For this review, use the dimensioned drawing (mm, ordinates from the lowest corner) and the shaded views. Give positions to 0.01 mm unless a question says otherwise; leave off trailing zeros. Order: outer loops, then holes, each group sorted by start corner. A loop starts at its lowest first (then second) coordinate and runs counter-clockwise, first axis right, second up. Notation, with made-up numbers: M 62,81 L 120,81 A10 cw 120,86 Z; hole C -32.5,23.25 d6. An arc over 180 degrees is marked long. Answer as CSV lines item,"result". Start each with the question number.
1. We need section B-B, the plane x = 114.3. Give the boundary of the cut face in (y, z) (3 decimals).
2. We need section C-C, the plane y = 50.8. Give the boundary of the cut face in (x, z) (3 decimals).
3. Clearance check with flat-ended pins moving along their axes: P1, Ø4, axis at x = 31.75, y = 50.8, coming from the -Z side; P2, Ø6, axis at x = 31.75, y = 12.7, coming from the +Z side (3 decimals). State where each tip first meets the part, or that it passes through.
4. We need section D-D, the plane y = 33. Give the boundary of the cut face in (x, z) (3 decimals), and give its area (3 significant figures).
5. We need section A-A, the plane x = 63.5. Give the boundary of the cut face in (y, z) (1 decimal), and give its area (3 significant figures).
6. For line 1 along Y through (x, z) = (12.7, 1.55); line 2 along X through (y, z) = (50.8, 1.1); line 3 along X through (y, z) = (12, 2.65), list the stretches that pass through material, from the lowest coordinate up.
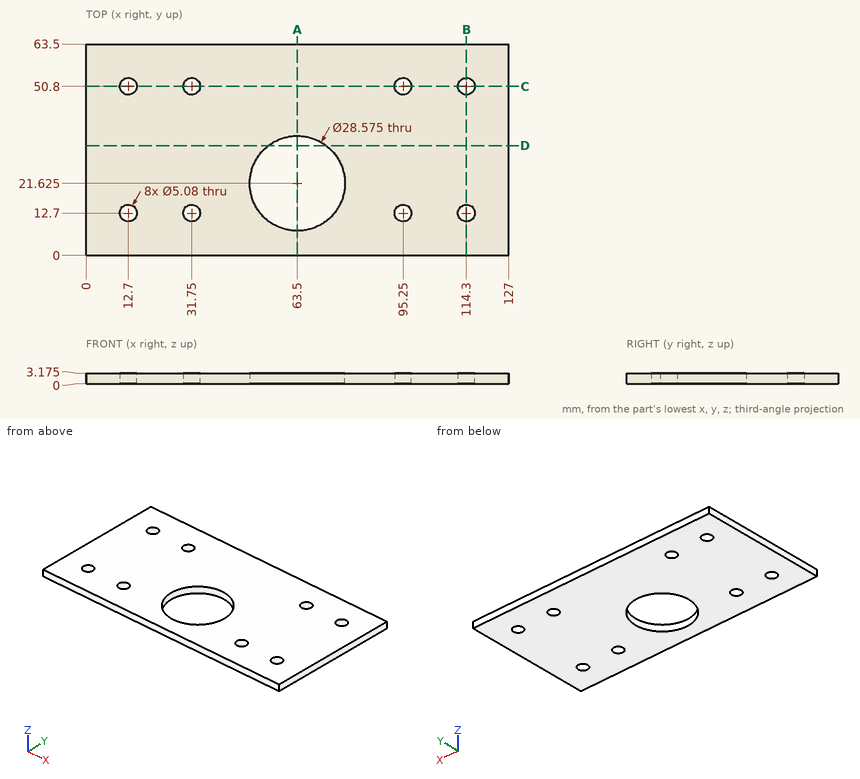
Result set:
1,outline,"M 0,0 L 10.16,0 L 10.16,3.175 L 0,3.175 Z; M 15.24,0 L 48.26,0 L 48.26,3.175 L 15.24,3.175 Z; M 53.34,0 L 63.5,0 L 63.5,3.175 L 53.34,3.175 Z"
2,outline,"M 0,0 L 10.16,0 L 10.16,3.175 L 0,3.175 Z; M 15.24,0 L 29.21,0 L 29.21,3.175 L 15.24,3.175 Z; M 34.29,0 L 92.71,0 L 92.71,3.175 L 34.29,3.175 Z; M 97.79,0 L 111.76,0 L 111.76,3.175 L 97.79,3.175 Z; M 116.84,0 L 127,0 L 127,3.175 L 116.84,3.175 Z"
3,P1,"through"
3,P2,"z = 3.175"
4,outline,"M 0,0 L 54.855,0 L 54.855,3.175 L 0,3.175 Z; M 72.145,0 L 127,0 L 127,3.175 L 72.145,3.175 Z"
4,area,"348 mm2"
5,outline,"M 0,0 L 7.3,0 L 7.3,3.2 L 0,3.2 Z; M 35.9,0 L 63.5,0 L 63.5,3.2 L 35.9,3.2 Z"
5,area,"111 mm2"
6,line 1,"0 to 10.16, 15.24 to 48.26, 53.34 to 63.5"
6,line 2,"0 to 10.16, 15.24 to 29.21, 34.29 to 92.71, 97.79 to 111.76, 116.84 to 127"
6,line 3,"0 to 10.26, 15.14 to 29.31, 34.19 to 52.94, 74.06 to 92.81, 97.69 to 111.86, 116.74 to 127"
